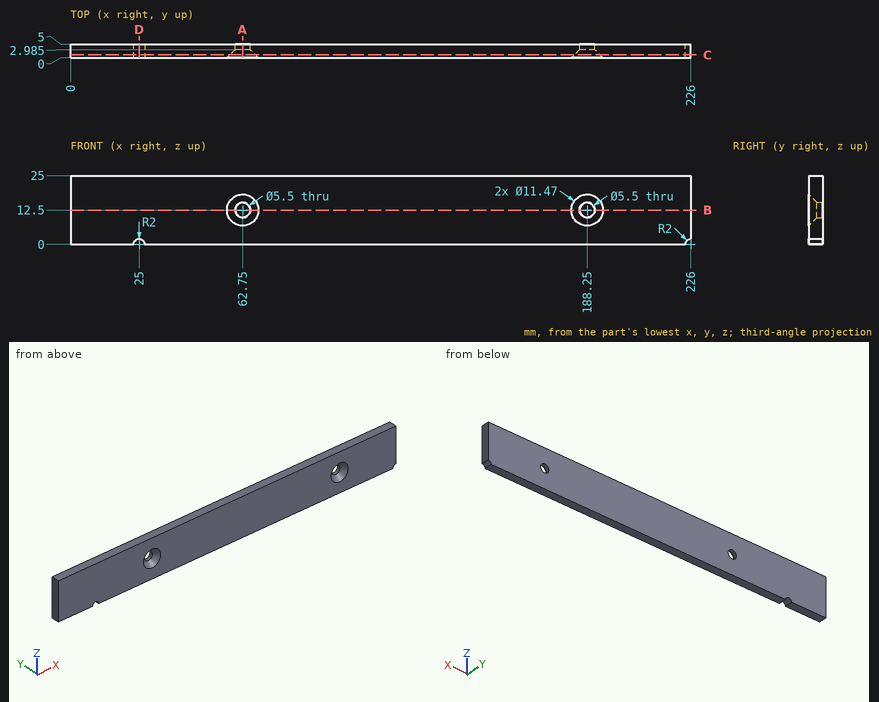
Here's the drawing with two shaded views (mm, measured from the low corner). I have some questions. Round coordinates to 2 decimals unless told otherwise and drop trailing zeros. Loops run counter-clockwise (first coordinate to the right, second up) from the corner with the lowest first, then second, coordinate; pieces in that order, holes last. Notation, with made-up numbers: (41, 15.25) - (57, 15.25) arc R20 cw to (57, 40.25) - close; hole circle Ø7 at (-34.5, 54). An arc over 180 degrees is marked (long way). Write item = value, one per line.
1) Imagine slicing it at D-D (x = 25). Please give me the cut outline in (y, z).
Computed:
outline = (0, 2) - (5, 2) - (5, 25) - (0, 25) - close
2) I'm going to push flat-ended pins straight in: P1, Ø7, axis at x = 188.25, z = 12.5, coming from the -Y side (3 decimals); P2, Ø9, axis at x = 62.75, z = 12.5, coming from the -Y side (3 decimals). Where does each tip first touch, or does it pass through?
Computed:
P1 = 2.235
P2 = 1.235
3) Imagine slicing it at B-B (z = 12.5). Please give me the cut outline in (x, y) (3 decimals), and give its area (3 significant figures).
Computed:
outline = (0, 0) - (57.015, 0) - (60, 2.985) - (60, 5) - (0, 5) - close; (65.5, 2.985) - (68.485, 0) - (182.515, 0) - (185.5, 2.985) - (185.5, 5) - (65.5, 5) - close; (191, 2.985) - (193.985, 0) - (226, 0) - (226, 5) - (191, 5) - close
area = 1,060 mm2
4) Imagine slicing it at A-A (x = 62.75). Please give me the cut outline in (y, z) (3 decimals).
Computed:
outline = (0, 0) - (5, 0) - (5, 9.75) - (2.985, 9.75) - (0, 6.765) - close; (0, 18.235) - (2.985, 15.25) - (5, 15.25) - (5, 25) - (0, 25) - close
5) I need wall thicknesses on line 1 along Z through (x, y) = (62.75, 4.1); line 2 along X through (y, z) = (2.8, 14.75); line 3 along X through (y, z) = (2.9, 11). Which ranges of each line are inside material? Lowest first, please. Write a range as from..to.
Computed:
line_1 = 0..9.75, 15.25..25
line_2 = 0..60.87, 64.63..186.37, 190.13..226
line_3 = 0..60.34, 65.16..185.84, 190.66..226
6) Imagine slicing it at C-C (y = 1). Please give me the cut outline in (x, z) (3 decimals).
Computed:
outline = (0, 0) - (23, 0) arc R2 cw to (27, 0) - (224, 0) arc R2 cw to (226, 2) - (226, 25) - (0, 25) - close; hole circle Ø9.47 at (62.75, 12.5); hole circle Ø9.47 at (188.25, 12.5)
